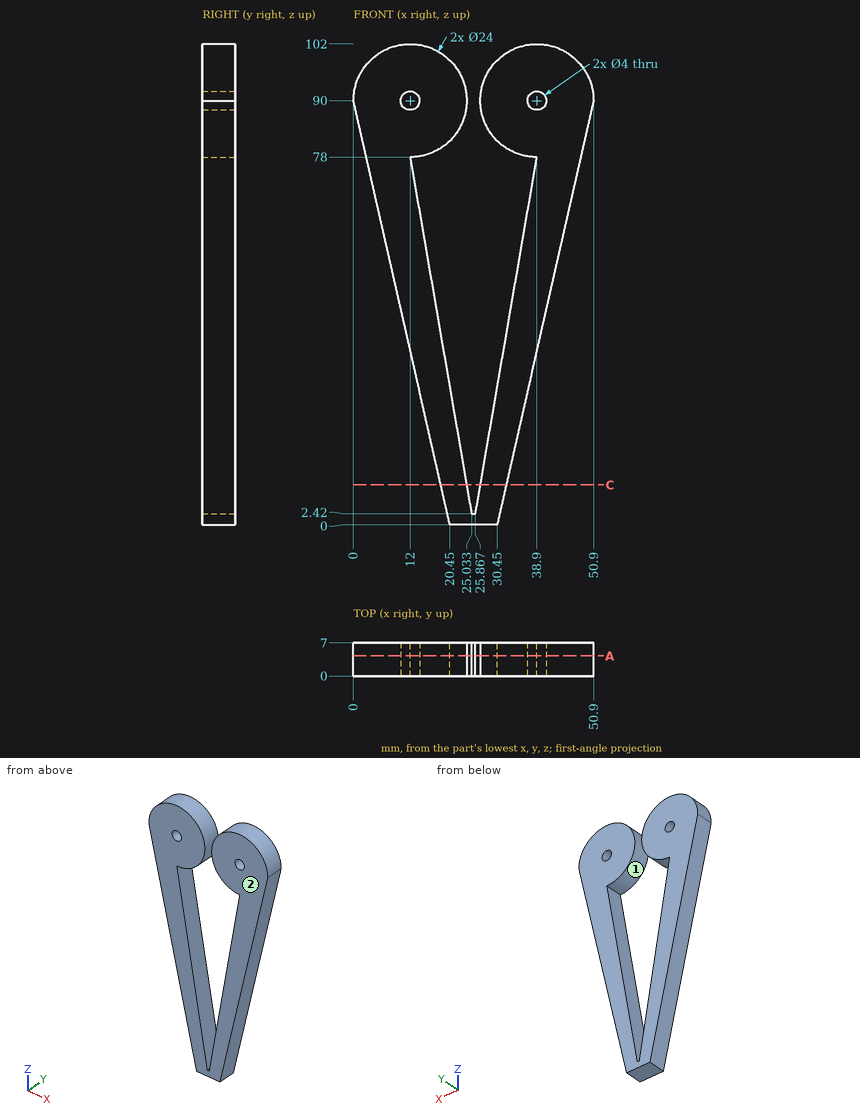
Design review of the part shown in the three views and the two pictorial views. Dimensions are in mm from the part's minimum x, y and z. Give positions to 0.01 mm unless a question says otherwise; leave off trailing zeros. Loops run counter-clockwise (first coordinate to the right, second up) from the corner with the lowest first, then second, coordinate; pieces in that order, holes last. Notation, with made-up numbers: (88, 54.25) - (136, 54.25) arc R22 cw to (136, 75.25) - close; hole circle Ø4 at (53, 45). An arc over 180 degrees is marked (long way). Answer as a JSON object with one key per item and string values.
Q1. Insertion check: pin 1 (3 mm diameter, centred on x = 12, z = 90, fed in from -Y). The pin has a flat end and moves straight along its axis. Give the tip position at first contact, or say it passes through.
Worked out:
{"pin 1": "passes through"}
Q2. Mouldability with a two-part tool opening along Z and no side actions: class the marked faces 1 and 2 as +Z half, -Z half, draft (parallel to the pull), parting line (faces both ways), or undercut.
Worked out:
{"face 1": "undercut", "face 2": "draft"}
Q3. Add section A-A on y = 4.25. State the section outline as (x, z) points, plus the area to 3 significant figures.
Worked out:
{"outline": "(0, 90) - (20.45, 0) - (30.45, 0) - (50.9, 90) arc R12 ccw (long way) to (38.9, 78) - (25.87, 2.42) - (25.03, 2.42) - (12, 78) arc R12 ccw (long way) to start; hole circle Ø4 at (12, 90); hole circle Ø4 at (38.9, 90)", "area": "2,020 mm^2"}
Q4. To check wall thickness, follow line 1 along X through (y, z) = (3.5, 90); line 2 along X through (y, z) = (5, 83) (1 decimal); line 3 along X through (y, z) = (3.25, 15). State the ranges of each line that lie inside material, in increasing order.
Worked out:
{"line 1": "x = 0 to 10, 14 to 24, 26.9 to 36.9, 40.9 to 50.9", "line 2": "x = 1.6 to 21.7, 29.2 to 49.3", "line 3": "x = 17.04 to 22.86, 28.04 to 33.86"}
Q5. Add section C-C on z = 8.5. State the section outline as (x, y) points (1 decimal).
Worked out:
{"outline": "(18.5, 0) - (24, 0) - (24, 7) - (18.5, 7) - close; (26.9, 0) - (32.4, 0) - (32.4, 7) - (26.9, 7) - close"}
